Model file for the job. Use its own axes, mm. A direction names the side the tool comes from. Give positions to 0.01 mm unless a question says otherwise; leave off trailing zeros. Write each loop counter-clockwise with the first axis right and the second up, starting at its lowest first coordinate (ties: lowest second). Pieces come first, ordered by that corner, then holes.
```python
from build123d import *

# Parameters (mm, degrees)
SKETCH1_W                = 50.8
SKETCH1_H                = 34.036
BOSS_EXTRUDE1_DEPTH      = 1.5875
CHAMFER2_SIZE            = 3.175
CUT_EXTRUDE1_DEPTH       = 3.175
SKETCH7_R                = 8.255
CUT_EXTRUDE3_DEPTH       = 3.175
SKETCH8_R                = 8.255
CUT_EXTRUDE4_DEPTH       = 3.175
SKETCH9_R                = 0.8
CUT_EXTRUDE5_DEPTH       = 3.175
SKETCH_1_W               = 50.8
SKETCH_1_H               = 8.7
CUT_EXTRUDE_1_DEPTH      = 10
SKETCH_2_W               = 50.8
SKETCH_2_H               = 3.18
EXTRUDE_1_DEPTH          = 19.05
CUT_EXTRUDE_2_DEPTH      = 10
SKETCH_3_R               = 2.5
CUT_EXTRUDE_3_DEPTH      = 10
SKETCH_5_R               = 5
SKETCH_5_R_2             = 2.5
EXTRUDE_2_DEPTH          = 6.6
CUT_EXTRUDE_4_REACH      = 38.887
CUT_EXTRUDE_4_END_RADIUS = 2.5
SKETCH_6_R               = 1.6
FILLET_1_R               = 1


with BuildPart() as part:
    # Sketch1 → Boss-Extrude1 (new, symmetric)
    with BuildSketch(Plane.XY):
        Rectangle(SKETCH1_W, SKETCH1_H)
    extrude(amount=BOSS_EXTRUDE1_DEPTH, both=True)

    # Chamfer2
    chamfer2_edges = [part.edges().sort_by_distance(p)[0] for p in [
        (-25.4, 17.018, 0),
        (25.4, 17.018, 0),
    ]]
    chamfer(chamfer2_edges, length=CHAMFER2_SIZE)

    # Sketch5 → Cut-Extrude1 (cut)
    with BuildSketch(Plane(origin=(0, 0, -1.5875), x_dir=(-1, 0, 0), z_dir=(0, 0, -1))):
        with BuildLine():
            Line((-5.969, 14.001104381), (-5.969, 17.018))
            Line((-5.969, 17.018), (5.969, 17.018))
            Line((5.969, 17.018), (5.969, 14.001104381))
            ThreePointArc((5.969, 14.001104381), (5.225051224, 12.205053157), (3.429, 11.461104381))
            Line((3.429, 11.461104381), (-3.429, 11.461104381))
            ThreePointArc((-3.429, 11.461104381), (-5.225051224, 12.205053157), (-5.969, 14.001104381))
        make_face()
    extrude(amount=-CUT_EXTRUDE1_DEPTH, mode=Mode.SUBTRACT)

    # Sketch7 → Cut-Extrude3 (cut)
    with BuildSketch(Plane(origin=(0, 0, -1.5875), x_dir=(-1, 0, 0), z_dir=(0, 0, -1))):
        with Locations((12.896, 6.34)):
            Circle(SKETCH7_R)
    extrude(amount=-CUT_EXTRUDE3_DEPTH, mode=Mode.SUBTRACT)

    # Sketch8 → Cut-Extrude4 (cut)
    with BuildSketch(Plane(origin=(0, 0, -1.5875), x_dir=(-1, 0, 0), z_dir=(0, 0, -1))):
        with Locations((-13.104, 6.34)):
            Circle(SKETCH8_R)
    extrude(amount=-CUT_EXTRUDE4_DEPTH, mode=Mode.SUBTRACT)

    # Sketch9 → Cut-Extrude5 (cut)
    with BuildSketch(Plane.XY.offset(1.5875)):
        with Locations((-21.306, 15.21)):
            Circle(SKETCH9_R)
        with Locations((21.514, 15.21)):
            Circle(SKETCH9_R)
        with Locations((21.514, -2.53)):
            Circle(SKETCH9_R)
        with Locations((-21.306, -2.53)):
            Circle(SKETCH9_R)
    extrude(amount=-CUT_EXTRUDE5_DEPTH, mode=Mode.SUBTRACT)

    # 草图1 → 切除-拉伸1 (cut)
    with BuildSketch(Plane.XY.offset(1.5875)):
        with Locations((0, -12.668)):
            Rectangle(SKETCH_1_W, SKETCH_1_H)
    extrude(amount=-CUT_EXTRUDE_1_DEPTH, mode=Mode.SUBTRACT)

    # 草图2 → 凸台-拉伸1 (add)
    with BuildSketch(Plane.XY.offset(1.5875)):
        with Locations((0, -6.728)):
            Rectangle(SKETCH_2_W, SKETCH_2_H)
    extrude(amount=EXTRUDE_1_DEPTH)

    # 草图4 → 切除-拉伸2 (cut)
    with BuildSketch(Plane(origin=(0, -5.138, 0), x_dir=(1, 0, 0), z_dir=(0, 1, 0))):
        with BuildLine():
            Line((-6, -4.0875), (6, -4.0875))
            ThreePointArc((6, -4.0875), (7.5, -5.5875), (6, -7.0875))
            Line((6, -7.0875), (-6, -7.0875))
            ThreePointArc((-6, -7.0875), (-7.5, -5.5875), (-6, -4.0875))
        make_face()
    extrude(amount=-CUT_EXTRUDE_2_DEPTH, mode=Mode.SUBTRACT)

    # 草图3 → 切除-拉伸3 (cut)
    with BuildSketch(Plane(origin=(0, -5.138, 0), x_dir=(1, 0, 0), z_dir=(0, 1, 0))):
        with Locations(Location((0, -12.6375, 0), (0, 0, 270))):
            Circle(SKETCH_3_R)
    extrude(amount=-CUT_EXTRUDE_3_DEPTH, mode=Mode.SUBTRACT)

    # 草图5 → 凸台-拉伸2 (add)
    with BuildSketch(Plane.XZ.offset(8.318)):
        with Locations(Location((0, 12.6375, 0), (0, 0, 270))):
            Circle(SKETCH_5_R)
        with Locations(Location((0, 12.6375, 0), (0, 0, 90))):
            Circle(SKETCH_5_R_2, mode=Mode.SUBTRACT)
    extrude(amount=EXTRUDE_2_DEPTH)

    # 切除-拉伸4: up to this cylinder (the profile starts outside it)
    cut_extrude_4_end = Plane(origin=(0, -11.518, 12.6375), z_dir=(0, 1, 0)) * Cylinder(CUT_EXTRUDE_4_END_RADIUS, 83.774, mode=Mode.PRIVATE)
    # 草图6 → 切除-拉伸4 (cut, up to the surface)
    with BuildSketch(Plane.XY, mode=Mode.PRIVATE) as cut_extrude_4_sk1:
        with Locations(Location((0, -11.518, 0), (0, 0, 180))):
            Circle(SKETCH_6_R)
    cut_extrude_4_tool1 = extrude(cut_extrude_4_sk1.sketch, amount=CUT_EXTRUDE_4_REACH, mode=Mode.PRIVATE) - cut_extrude_4_end
    add(cut_extrude_4_tool1.solids().sort_by_distance((0, -11.518, 0))[0], mode=Mode.SUBTRACT)

    # 圆角1
    fillet_1_edges = [part.edges().sort_by_distance(p)[0] for p in [
        (0, -8.318, 17.6375),
    ]]
    fillet(fillet_1_edges, radius=FILLET_1_R)


solid = part.part
```
1. Pin check, flat tips, straight feed: P1, Ø1.8, axis at x = 21.514, y = 15.21, coming from the +Z side; P2, Ø12, axis at x = 10, z = 4.5, coming from the -Y side; P3, Ø2.5, axis at y = 15.5, z = 0.5, coming from the +X side; P4, Ø10, axis at y = -3, z = 5.5, coming from the -X side. Stop position of each tip, or through.
Calculated:
P1: stops at z = 1.59
P2: stops at y = -8.32
P3: stops at x = 24.99
P4: stops at x = -25.4
2. Pull direction Z, two halves, no side cores. Call faces 1 (the flat face through (0, 6, 1.588)), 2 (the flat face through (0, -7, 7.088)), 3 (the flat face through (0, -7, 4.088)), 4 (the cylindrical face through (5.21, 12.19, -0.02)): +Z half, -Z half, draft (parallel to the pull), parting line (faces both ways), or undercut.
Calculated:
face 1: +Z half
face 2: undercut
face 3: undercut
face 4: draft
3. Slice it at D-D, the plane x = 19.5. Write the cut outline in (y, z).
Calculated:
outline: (-8.32, -1.59) - (1.12, -1.59) - (1.12, 1.59) - (-5.14, 1.59) - (-5.14, 20.64) - (-8.32, 20.64) - close; (11.56, -1.59) - (17.02, -1.59) - (17.02, 1.59) - (11.56, 1.59) - close
4. Which spindle directions (+Z, -Z, +X, -X, +Y, -Y) get a long thin tool onto all of the face, cutting with end or side? Do faces 5 (the flat face through (5.969, 15, 0)), 6 (the cylindrical face through (-7.5, -6.7, 5.6)), 7 (the cylindrical face through (-1.526, -11.999, 9.155)), 8 (the cylindrical face through (-6.345, 1.317, -0.022)). Say none if no direction does.
Calculated:
face 5: +Z, -Z, +Y
face 6: +Y, -Y
face 7: -Z
face 8: +Z, -Z
5. Slice it at C-C, the plane y = -7. Write the cut outline in (x, z).
Calculated:
outline: (-25.4, -1.59) - (25.4, -1.59) - (25.4, 20.64) - (-25.4, 20.64) - close; hole (-6, 4.09) - (6, 4.09) arc R1.5 ccw to (6, 7.09) - (-6, 7.09) arc R1.5 ccw to start; hole circle Ø5 at (0, 12.64)
6. Slice it at B-B, the plane z = 0. Write the cut outline in (x, y) (3 decimals).
Calculated:
outline: (-25.4, -8.318) - (25.4, -8.318) - (25.4, 13.843) - (22.225, 17.018) - (5.969, 17.018) - (5.969, 14.001) arc R2.54 cw to (3.429, 11.461) - (-3.429, 11.461) arc R2.54 cw to (-5.969, 14.001) - (-5.969, 17.018) - (-22.225, 17.018) - (-25.4, 13.843) - close; hole circle Ø1.6 at (-21.306, -2.53); hole circle Ø1.6 at (-21.306, 15.21); hole circle Ø16.51 at (-12.896, 6.34); hole circle Ø16.51 at (13.104, 6.34); hole circle Ø1.6 at (21.514, -2.53); hole circle Ø1.6 at (21.514, 15.21)
7. Probe probe 1 along X at (y, z) = (-2, -0.5); probe 2 along Y at (x, z) = (0, 8.7); probe 3 along Z at (x, y) = (0.5, -2). List the from-to ranges inside material, lowest first.
Calculated:
probe 1: x = -25.4 to -21.91, -20.71 to 20.91, 22.11 to 25.4
probe 2: y = -14.92 to -13.12, -9.92 to -5.14
probe 3: z = -1.59 to 1.59
8. Slice it at A-A, the plane y = -2.53. Write the cut outline in (x, z).
Calculated:
outline: (-25.4, -1.59) - (-22.11, -1.59) - (-22.11, 1.59) - (-25.4, 1.59) - close; (-20.51, -1.59) - (20.71, -1.59) - (20.71, 1.59) - (-20.51, 1.59) - close; (22.31, -1.59) - (25.4, -1.59) - (25.4, 1.59) - (22.31, 1.59) - close
